Source: CAD feature listing. Evaluate the final solid. Frame: model axes, mm. A direction names the side the tool comes from. Give positions to 0.01 mm unless a question says otherwise; leave off trailing zeros. Loops run counter-clockwise (first coordinate to the right, second up) from the corner with the lowest first, then second, coordinate; pieces in that order, holes last. Notation, with made-up numbers: (89.25, 21.5) -> (118.25, 21.5) arc R18 ccw to (118.25, 56.5) -> close; hole circle Ø10 at (22, 83). An arc over 180 degrees is marked (long way). Put each result on its own line as item: value.
```python
from build123d import *

# Parameters (mm, degrees)
SKETCH_1_W      = 20
SKETCH_1_H      = 27
SKETCH_1_R      = 1.1
SKETCH_1_R_2    = 4
EXTRUDE_1_DEPTH = 4.8
FILLET_3_R      = 2.5
FILLET_4_R      = 2.5
SKETCH_2_W      = 6.666666666
SKETCH_2_H      = 1.6
EXTRUDE_2_DEPTH = 3


with BuildPart() as part:
    # 草图1 → 凸台-拉伸1 (new body)
    with BuildSketch(Plane(origin=(0, 0, 0), x_dir=(1, 0, 0), z_dir=(0, 1, 0))):
        with Locations((0, -3.5)):
            Rectangle(SKETCH_1_W, SKETCH_1_H)
        with Locations(Location((7.424621202, 7.424621202, 0), (0, 0, 270))):
            Circle(SKETCH_1_R, mode=Mode.SUBTRACT)
        with Locations(Location((7.424621202, -7.424621202, 0), (0, 0, 270))):
            Circle(SKETCH_1_R, mode=Mode.SUBTRACT)
        with Locations(Location((-7.424621202, -7.424621202, 0), (0, 0, 270))):
            Circle(SKETCH_1_R, mode=Mode.SUBTRACT)
        with Locations(Location((-7.424621202, 7.424621202, 0), (0, 0, 270))):
            Circle(SKETCH_1_R, mode=Mode.SUBTRACT)
        with Locations(Location((0, 0, 0), (0, 0, 270))):
            Circle(SKETCH_1_R_2, mode=Mode.SUBTRACT)
    extrude(amount=EXTRUDE_1_DEPTH)

    # 圆角3
    fillet_3_edges = [part.edges().sort_by_distance(p)[0] for p in [
        (-10, 2.4, -10),
    ]]
    fillet(fillet_3_edges, radius=FILLET_3_R)

    # 圆角4
    fillet_4_edges = [part.edges().sort_by_distance(p)[0] for p in [
        (10, 2.4, -10),
    ]]
    fillet(fillet_4_edges, radius=FILLET_4_R)

    # 草图2 → 凸台-拉伸2 (add)
    with BuildSketch(Plane.XY.offset(17)):
        with Locations((0, 2.4)):
            Rectangle(SKETCH_2_W, SKETCH_2_H)
    extrude(amount=EXTRUDE_2_DEPTH)


solid = part.part
```
(1) Section C-C on y = 1.3. Return loops of the section in (x, z), then the cut area to 3 significant figures.
Calculated:
outline: (-10, -7.5) arc R2.5 ccw to (-7.5, -10) -> (7.5, -10) arc R2.5 ccw to (10, -7.5) -> (10, 17) -> (-10, 17) -> close; hole circle Ø2.2 at (-7.42, -7.42); hole circle Ø2.2 at (-7.42, 7.42); hole circle Ø8 at (0, 0); hole circle Ø2.2 at (7.42, -7.42); hole circle Ø2.2 at (7.42, 7.42)
area: 472 mm²
(2) Section B-B on z = 0. Return loops of the section in (x, y), then the cut area to 3 significant figures.
Calculated:
outline: (-10, 0) -> (-4, 0) -> (-4, 4.8) -> (-10, 4.8) -> close; (4, 0) -> (10, 0) -> (10, 4.8) -> (4, 4.8) -> close
area: 57.6 mm²
(3) Line query: probe 1 along Z at (x, y) = (7.5, 2.2); probe 2 along Z at (x, y) = (-0.25, 3.55); probe 3 along Z at (x, y) = (-7, 1.75). Output: solid intervals per line, ascending. Write a range as from..to.
Calculated:
probe 1: z = -10..-8.52, -6.33..6.33, 8.52..17
probe 2: z = -10..-3.99, 3.99..17
probe 3: z = -10..-8.44, -6.41..6.41, 8.44..17
(4) Section A-A on x = 0. Return loops of the section in (y, z).
Calculated:
outline: (0, -10) -> (4.8, -10) -> (4.8, -4) -> (0, -4) -> close; (0, 4) -> (4.8, 4) -> (4.8, 17) -> (3.2, 17) -> (3.2, 20) -> (1.6, 20) -> (1.6, 17) -> (0, 17) -> close
(5) First-contact query: P1, Ø1.5, axis at x = 1.5, z = 19, coming from the +Y side; P2, Ø0.8, axis at y = 2.5, z = 18.5, coming from the -X side; P3, Ø1.3, axis at y = 2, z = 18.5, coming from the +X side. Flat tips, straight axial feed; report the tip coordinate or a pass-through.
Calculated:
P1: stops at y = 3.2
P2: stops at x = -3.33
P3: stops at x = 3.33
(6) Section D-D on x = 6.75. Return loops of the section in (y, z), then the cut area to 3 significant figures.
Calculated:
outline: (0, -10) -> (4.8, -10) -> (4.8, -8.29) -> (0, -8.29) -> close; (0, -6.56) -> (4.8, -6.56) -> (4.8, 6.56) -> (0, 6.56) -> close; (0, 8.29) -> (4.8, 8.29) -> (4.8, 17) -> (0, 17) -> close
area: 113 mm²
(7) Reachability of faces 1 (the flat face through (0, 1.6, 18)), 2 (the cylindrical face through (9.248, 2.434, -9.287)), 3 (the flat face through (0, 3.2, 18)), 4 (the flat face through (-3.333, 2, 18)) from +Z, -Z, +X, -X, +Y, -Y: full face, straight path, thin tool, end or side. Return the list, or none.
Calculated:
face 1: +Z, +X, -X, -Y
face 2: -Z, +X, +Y, -Y
face 3: +Z, +X, -X, +Y
face 4: +Z, -X, +Y, -Y
(8) Draft query along X for faces 5 (the flat face through (0, 2, -10)), 6 (the flat face through (3.333, 2, 18)), 7 (the cylindrical face through (-8.4, 2.37, 7.93)). Return one class per face: released by +X, released by -X, zero draft, split by the parting line, or undercut.
Calculated:
face 5: zero draft
face 6: released by +X
face 7: undercut
